Geometry check sheet. Reference: the model listing, model coordinates, mm. Face numbers are marked on the shaded views. A direction names the side the tool comes from. Coordinates: 2 decimals unless noted, no trailing zeros. Loops run counter-clockwise (first coordinate to the right, second up) from the corner with the lowest first, then second, coordinate; pieces in that order, holes last. Notation, with made-up numbers: (48, -34.75) -> (97, -34.75) arc R23 cw to (97, 1.25) -> close; hole circle Ø6 at (-33.5, -7). An arc over 180 degrees is marked (long way). Answer as a JSON object with one key per item and string values.
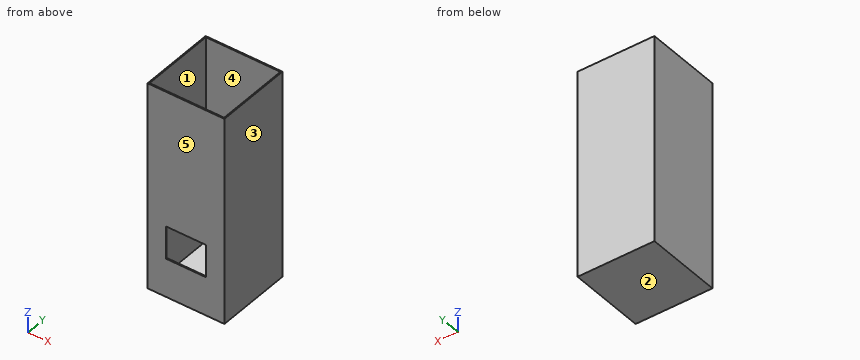
from build123d import *

# Parameters (mm, degrees)
F0_W     = 388
F0_H     = 388
F1_DEPTH = 6
F0_W_2   = 400
F0_H_2   = 400
F2_DEPTH = 1080
F3_W     = 210
F3_H     = 170
F4_DEPTH = 25


with BuildPart() as f1:
    # F0 (on Top) → F1 (new body)
    with BuildSketch(Plane.XY):
        Rectangle(F0_W, F0_H)
    extrude(amount=F1_DEPTH)

    # F0 (on Top) → F2 (join)
    with BuildSketch(Plane.XY):
        Rectangle(F0_W_2, F0_H_2)
        Rectangle(F0_W, F0_H, mode=Mode.SUBTRACT)
    extrude(amount=F2_DEPTH)

    # F3 (on face) → F4 (cut)
    with BuildSketch(Plane.XZ.offset(200)):
        with Locations((0, 286.11201)):
            Rectangle(F3_W, F3_H)
    extrude(amount=-F4_DEPTH, mode=Mode.SUBTRACT)


solid = f1.part
1. Tool access check on the marked faces 4 and 5. Record the directions out of +Z, -Z, +X, -X, +Y, -Y that give a thin tool (end or side, any length) a straight path to the whole face; none if there is none.
Evaluation:
{"face 4": "+Z", "face 5": "+Z, -Z, +X, -X, -Y"}
2. Section check B-B, the plane y = 113. Record the boundary of the cut face in (x, z), then the cut area to 3 significant figures.
Evaluation:
{"outline": "(-200, 0) -> (200, 0) -> (200, 1080) -> (194, 1080) -> (194, 6) -> (-194, 6) -> (-194, 1080) -> (-200, 1080) -> close", "area": "15,300 mm^2"}
3. Thickness scan on probe 1 along Y at (x, z) = (56, 944.5); probe 2 along Z at (x, y) = (-89.5, 157). Record the ranges inside material, lowest first. Write a range as from..to.
Evaluation:
{"probe 1": "y = -200..-194, 194..200", "probe 2": "z = 0..6"}
4. Section check C-C, the plane z = 399. Record the boundary of the cut face in (x, y), then the cut area to 3 significant figures.
Evaluation:
{"outline": "(-200, -200) -> (200, -200) -> (200, 200) -> (-200, 200) -> close; hole (-194, -194) -> (194, -194) -> (194, 194) -> (-194, 194) -> close", "area": "9,460 mm^2"}
5. Depth check by flat-ended pin: P1, Ø4, axis at x = -119.5, y = -104, coming from the +Z side. Enter the tip coordinate at first touch or a pass-through.
Evaluation:
{"P1": "stops at z = 6"}
6. Mould release check, pull along X, two halves, no side actions. Record for the marked faces 1, 2 and 3: released by +X, released by -X, zero draft, split by the parting line, or undercut.
Evaluation:
{"face 1": "undercut", "face 2": "zero draft", "face 3": "released by +X"}
7. Section check A-A, the plane x = 29.5. Record the boundary of the cut face in (y, z).
Evaluation:
{"outline": "(-200, 0) -> (200, 0) -> (200, 1080) -> (194, 1080) -> (194, 6) -> (-194, 6) -> (-194, 201.11) -> (-200, 201.11) -> close; (-200, 371.11) -> (-194, 371.11) -> (-194, 1080) -> (-200, 1080) -> close"}
